Can you work these out from the model? Positions are in its coordinate system, mm. A direction names the side the tool comes from. Coordinates: 2 decimals unless noted, no trailing zeros. Order: outer loops, then holes, each group sorted by start corner. A loop starts at its lowest first (then second) coordinate and runs counter-clockwise, first axis right, second up. Notation, with made-up numbers: (-11, 41) -> (30, 41) arc R17 cw to (30, 74) -> close; hole circle Ø4 at (-4, 70.25). An arc over 180 degrees is marked (long way). Use a Markdown table: item, result. Add a question column.
1. For pin 1 Ø2.5 at (x, y) = (22.86, 16.51) entering from +Z; pin 2 Ø4.5 at (x, y) = (21.5, 15.5) entering from +Z, each with a flat end and sliding along its axis, tell me the tip position at first contact or that it passes through.
2. Suppose I cut it at A-A, the plane y = -16.51. List the corners of the cut face in (x, z) for me.
3. Suppose I cut it at D-D, the plane x = -17.5. List the corners of the cut face in (y, z) for me.
4. If I drill on line 1 along Y through (x, z) = (-22.86, 0.3); line 2 along Y through (x, z) = (22, 1.5); line 3 along Z through (x, y) = (18, -15.5), over which ranges is the centre line in solid material (lowest first)? Write a range as from..to.
5. For faces 5 (the flat face through (0, 0, 11.938)), 6 (the cylindrical face through (-18.87, -11.57, 6.84)), which set-ups out of +Z, -Z, +X, -X, +Y, -Y let a thin tool reach every point of the face, with its end or its side?
6. Suppose I cut it at B-B, the plane x = -22.86. List the corners of the cut face in (y, z) for me, then the cut area to 3 significant figures.
7. Suppose I cut it at C-C, the plane z = 10.25. List the corners of the cut face in (x, y) for me.
8. We'd pull the mould along Y, two halves only. Please class faces 1 (the flat face through (0, 0, 0)), 2 (the flat face through (0, 18.669, 6)), 3 (the cylindrical face through (24.56, -16.44, 0.78)), 4 (the cylindrical face through (-21.16, -16.44, 0.78)): pulls with the +Y half, pulls with the -Y half, needs draft (parallel to the pull), parting line crosses it, or undercut.
```python
from build123d import *

# Parameters (mm, degrees)
SKETCH1_W                = 52.832
SKETCH1_H                = 37.338
BOSS_EXTRUDE1_DEPTH      = 11.938
M3_CLEARANCE_HOLE1_D     = 3.4
M3_CLEARANCE_HOLE1_DEPTH = 11.938
SKETCH4_R                = 6.35
CUT_EXTRUDE1_DEPTH       = 10.3505


with BuildPart() as part:
    # Sketch1 → Boss-Extrude1 (new body)
    with BuildSketch(Plane.XY):
        Rectangle(SKETCH1_W, SKETCH1_H)
    extrude(amount=BOSS_EXTRUDE1_DEPTH)

    # M3 Clearance Hole1
    with Locations(Plane.XY.offset(11.938)):
        with Locations((-22.86, 16.51), (22.86, -16.51), (22.86, 16.51), (-22.86, -16.51)):
            Hole(M3_CLEARANCE_HOLE1_D / 2, depth=M3_CLEARANCE_HOLE1_DEPTH)

    # Sketch4 → Cut-Extrude1 (cut)
    with BuildSketch(Plane.XY.offset(11.938)):
        with Locations((-22.86, 16.51)):
            Circle(SKETCH4_R)
        with Locations((-22.86, -16.51)):
            Circle(SKETCH4_R)
        with Locations((22.86, 16.51)):
            Circle(SKETCH4_R)
        with Locations((22.86, -16.51)):
            Circle(SKETCH4_R)
    extrude(amount=-CUT_EXTRUDE1_DEPTH, mode=Mode.SUBTRACT)


solid = part.part
```
Worked out:
| question | item | result |
|---|---|---|
| 1 | pin 1 | passes through |
| 1 | pin 2 | stops at z = 1.59 |
| 2 | outline | (-26.42, 0) -> (-24.56, 0) -> (-24.56, 1.59) -> (-26.42, 1.59) -> close; (-21.16, 0) -> (21.16, 0) -> (21.16, 1.59) -> (16.51, 1.59) -> (16.51, 11.94) -> (-16.51, 11.94) -> (-16.51, 1.59) -> (-21.16, 1.59) -> close; (24.56, 0) -> (26.42, 0) -> (26.42, 1.59) -> (24.56, 1.59) -> close |
| 3 | outline | (-18.67, 0) -> (18.67, 0) -> (18.67, 1.59) -> (13.11, 1.59) -> (13.11, 11.94) -> (-13.11, 11.94) -> (-13.11, 1.59) -> (-18.67, 1.59) -> close |
| 4 | line 1 | y = -18.67..-18.21, -14.81..14.81, 18.21..18.67 |
| 4 | line 2 | y = -18.67..-17.98, -15.04..15.04, 17.98..18.67 |
| 4 | line 3 | z = 0..1.59 |
| 5 | face 5 | +Z, +X, -X, +Y, -Y |
| 5 | face 6 | +Z |
| 6 | outline | (-18.67, 0) -> (-18.21, 0) -> (-18.21, 1.59) -> (-18.67, 1.59) -> close; (-14.81, 0) -> (14.81, 0) -> (14.81, 1.59) -> (10.16, 1.59) -> (10.16, 11.94) -> (-10.16, 11.94) -> (-10.16, 1.59) -> (-14.81, 1.59) -> close; (18.21, 0) -> (18.67, 0) -> (18.67, 1.59) -> (18.21, 1.59) -> close |
| 6 | area | 259 mm² |
| 7 | outline | (-26.42, -11.25) arc R6.35 cw to (-16.89, -18.67) -> (16.89, -18.67) arc R6.35 cw to (26.42, -11.25) -> (26.42, 11.25) arc R6.35 cw to (16.89, 18.67) -> (-16.89, 18.67) arc R6.35 cw to (-26.42, 11.25) -> close |
| 8 | face 1 | needs draft |
| 8 | face 2 | pulls with the +Y half |
| 8 | face 3 | undercut |
| 8 | face 4 | undercut |
